Part print with two shaded views. Sizes in mm from the minimum x, y, z corner. A direction names the side the tool comes from. Give positions to 0.01 mm unless a question says otherwise; leave off trailing zeros. Loops run counter-clockwise (first coordinate to the right, second up) from the corner with the lowest first, then second, coordinate; pieces in that order, holes last. Notation, with made-up numbers: M 3,3 L 38,3 A15 ccw 38,16 Z; hole C -5,-35.5 d5. An arc over 180 degrees is marked long. Answer as a JSON object with one key per item and string values. Group by question number.
1. Slice it at A-A (y = 36.5). List the corners of the cut face in (x, z).
2. 3-axis set-ups, long thin cutter, end or side, ignore diameter. For the marked faces 1 and 2: which of +Z, -Z, +X, -X, +Y, -Y reach the whole face in a straight line?
3. Slice it at D-D (x = 21). List the corners of the cut face in (y, z), then the cut area to 3 significant figures.
4. Drop flat-ended pins along their axis: pin 1 Ø2.5 at (x, y) = (36.5, 5.5) entering from +Z; pin 2 Ø10 at (x, y) = (35, 15.5) entering from +Z; pin 3 Ø3.5 at (x, y) = (5.5, 5.5) entering from +Z. Give the stop position or say it passes through.
5. Slice it at B-B (z = 31). List the corners of the cut face in (x, y).
6. Drill centre lines: line 1 along Y through (x, z) = (5.5, 26.5); line 2 along X through (y, z) = (36, 11); line 3 along Z through (x, y) = (12, 26). Where is each one in solid material? Low to high. Write a range as [from, to].
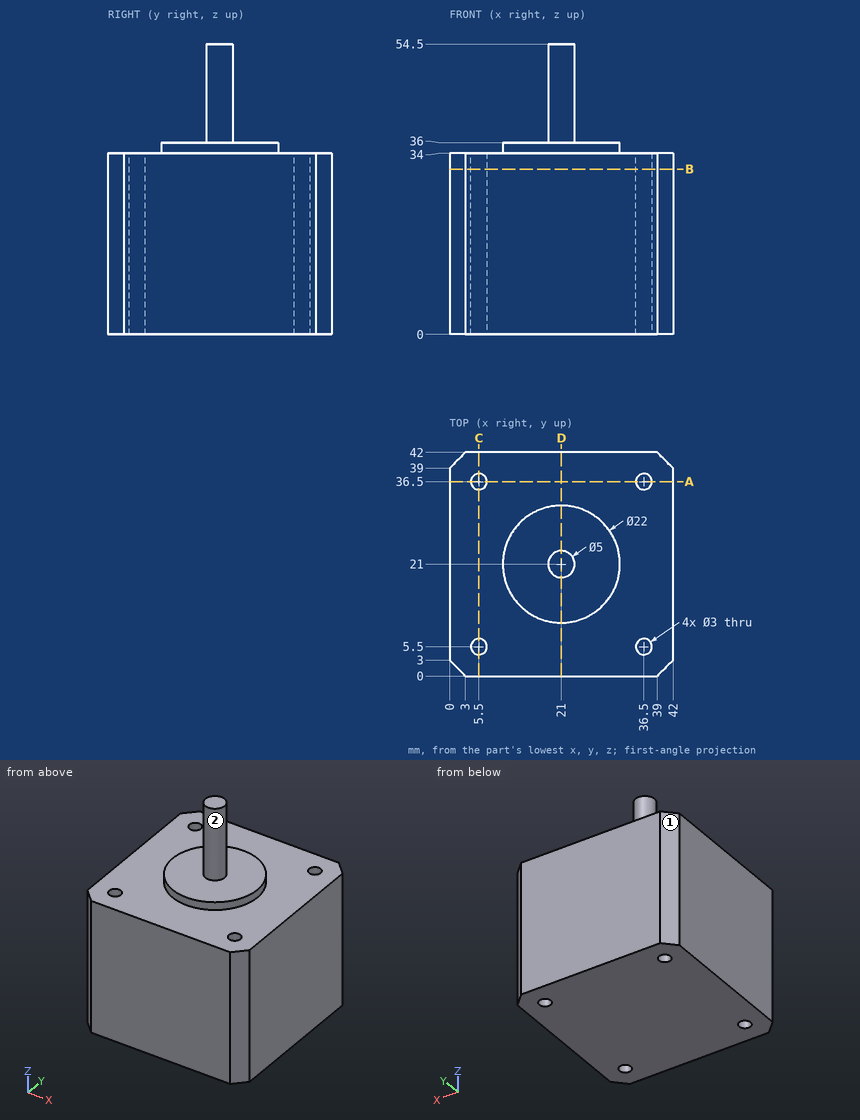
Established:
{
 "1": {"outline": "M 0,0 L 4,0 L 4,34 L 0,34 Z; M 7,0 L 35,0 L 35,34 L 7,34 Z; M 38,0 L 42,0 L 42,34 L 38,34 Z"},
 "2": {"face 1": "+Z, -Z, -X, +Y", "face 2": "+Z"},
 "3": {"outline": "M 0,0 L 42,0 L 42,34 L 32,34 L 32,36 L 23.5,36 L 23.5,54.5 L 18.5,54.5 L 18.5,36 L 10,36 L 10,34 L 0,34 Z", "area": "1,560 mm^2"},
 "4": {"pin 1": "passes through", "pin 2": "stops at z = 36", "pin 3": "stops at z = 34"},
 "5": {"outline": "M 0,3 L 3,0 L 39,0 L 42,3 L 42,39 L 39,42 L 3,42 L 0,39 Z; hole C 5.5,5.5 d3; hole C 5.5,36.5 d3; hole C 36.5,5.5 d3; hole C 36.5,36.5 d3"},
 "6": {"line 1": "y = [0, 4], [7, 35], [38, 42]", "line 2": "x = [0, 4.09], [6.91, 35.09], [37.91, 42]", "line 3": "z = [0, 36]"}
}
